from build123d import *

# Parameters (mm, degrees)
SKETCH_1_R      = 3
EXTRUDE_1_DEPTH = 3


with BuildPart() as part:
    # 草图1 → 凸台-拉伸1 (new body)
    with BuildSketch(Plane.XY):
        with BuildLine():
            Line((8.44582472, 166.89164944), (15, 180))
            ThreePointArc((15, 180), (30, 189.270509831), (45, 180))
            Line((45, 180), (51.55417528, 166.89164944))
            ThreePointArc((51.55417528, 166.89164944), (57.859919157, 149.494795444), (60, 131.1145618))
            Line((60, 131.1145618), (60, 125.412430481))
            ThreePointArc((60, 125.412430481), (59.589066182, 121.379009336), (58.373151387, 117.511335106))
            ThreePointArc((58.373151387, 117.511335106), (50.063143822, 62.228284379), (70, 10))
            Line((70, 10), (70, 0))
            Line((70, 0), (60, 0))
            Line((60, 0), (0, 0))
            Line((0, 0), (0, 10))
            ThreePointArc((0, 10), (-10.668063464, 65.5572809), (0, 121.1145618))
            Line((0, 121.1145618), (0, 131.1145618))
            ThreePointArc((0, 131.1145618), (2.140080843, 149.494795444), (8.44582472, 166.89164944))
        make_face()
        with Locations((10, 10)):
            Circle(SKETCH_1_R, mode=Mode.SUBTRACT)
        with Locations((50, 10)):
            Circle(SKETCH_1_R, mode=Mode.SUBTRACT)
        with Locations((30, 180)):
            Circle(SKETCH_1_R, mode=Mode.SUBTRACT)
    extrude(amount=EXTRUDE_1_DEPTH)


solid = part.part
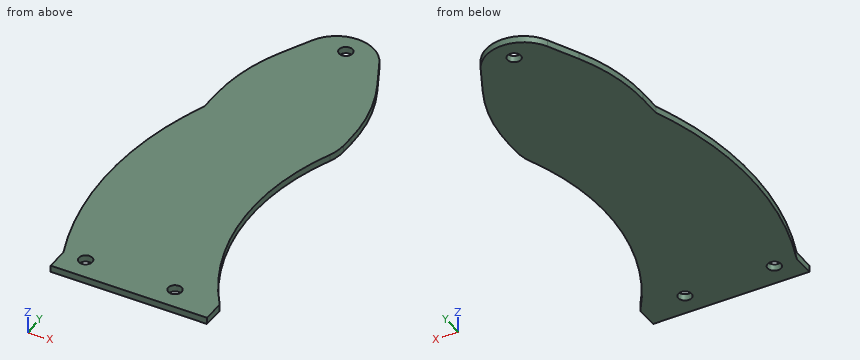
Geometry: final body of the model. Coordinates: model frame, mm. Give positions to 0.01 mm unless a question says otherwise; leave off trailing zeros. Loops run counter-clockwise (first coordinate to the right, second up) from the corner with the lowest first, then second, coordinate; pieces in that order, holes last. Notation, with made-up numbers: (30, 60.25) -> (76, 60.25) arc R27 cw to (76, 82.25) -> close; hole circle Ø4 at (-7, -4.75). An arc over 180 degrees is marked (long way). Put each result on its own line as item: value.
1. Cut plane C-C (y = 16.5). Return the cut outline in (x, z).
Taken from the geometry:
outline: (-2.42, 0) -> (65.68, 0) -> (65.68, 3) -> (-2.42, 3) -> close
2. Pin query (flat end, axial travel): P1, Ø0.9, axis at y = 3, z = 2, coming from the -X side; P2, Ø1, axis at x = 7, z = 2, coming from the +Y side; P3, Ø8, axis at x = 54.5, y = 66.5, coming from the +Z side. Return the tip coordinate at first contact, or that it passes through.
Taken from the geometry:
P1: stops at x = 0
P2: stops at y = 164.93
P3: passes through
3. Ray query, line 1 along Y through (x, z) = (10, 2.35); line 2 along X through (y, z) = (176, 0.75); line 3 along X through (y, z) = (29.5, 2.3). Return the intervals inside material, ascending. Write a range as [from, to].
Taken from the geometry:
line 1: y = [0, 7], [13, 170]
line 2: x = [13, 47]
line 3: x = [-6.27, 58.85]
4. Cut plane D-D (x = 19). Return the cut outline in (y, z).
Taken from the geometry:
outline: (0, 0) -> (185.16, 0) -> (185.16, 3) -> (0, 3) -> close
5. Cut plane B-B (z = 1.15). Return the cut outline in (x, y).
Taken from the geometry:
outline: (0, 0) -> (70, 0) -> (70, 10) arc R110 cw to (58.37, 117.51) arc R20 ccw to (60, 125.41) -> (60, 131.11) arc R80 ccw to (51.55, 166.89) -> (45, 180) arc R16.77 ccw to (15, 180) -> (8.45, 166.89) arc R80 ccw to (0, 131.11) -> (0, 121.11) arc R150 ccw to (0, 10) -> close; hole circle Ø6 at (10, 10); hole circle Ø6 at (30, 180); hole circle Ø6 at (50, 10)
6. Cut plane A-A (x = 30). Return the cut outline in (y, z).
Taken from the geometry:
outline: (0, 0) -> (177, 0) -> (177, 3) -> (0, 3) -> close; (183, 0) -> (189.27, 0) -> (189.27, 3) -> (183, 3) -> close
